Input: part model. Units: mm. Frame: model coordinates. A direction names the side the tool comes from. Give positions to 0.01 mm unless a question says otherwise; leave off trailing zeros. Loops run counter-clockwise (first coordinate to the right, second up) from the corner with the lowest first, then second, coordinate; pieces in that order, holes last. Notation, with made-up numbers: (74.25, 34.5) -> (83.25, 34.5) arc R9 cw to (83.25, 49.5) -> close; hole circle Ø8 at (-18.75, 11). An arc over 180 degrees is marked (long way). Answer as a JSON object with one key per item and string values. Group by question number.
Autodesk Inventor part; units mm, degrees
ref_plane "YZ Plane" through (0, 0, 0) normal (1, 0, 0) x (0, 1, 0)
ref_plane "XZ Plane" through (0, 0, 0) normal (0, 1, 0) x (-1, 0, 0)
ref_plane "XY Plane" through (0, 0, 0) normal (0, 0, 1) x (1, 0, 0)
sketch "Sketch1" plane through (0, 0, 0) normal (0, 1, 0) x (-1, 0, 0)
  line L0 (125, 0) -> (125, -63)
  line L1 (125, -63) -> (-4.2, -63)
  line L2 (-4.2, -63) -> (-4.2, 0)
  line L3 (-4.2, 0) -> (5.8, 0)
  line L4 (5.8, 0) -> (5.8, 40)
  line L5 (20.8, 40) -> (20.8, 0)
  line L6 (20.8, 0) -> (125, 0)
  line L7 (5.8, 40) -> (5.8, 70)
  line L8 (5.8, 70) -> (20.8, 70)
  line L9 (20.8, 70) -> (20.8, 40)
  line L10 (125, 0) -> (125, 20)
  line L11 (125, 20) -> (5.8, 20)
  line L12 (-4.2, -1.8) -> (-4.2, -60.8)
  line L13 (-4.2, 0) -> (5.8, 20)
  line L14 (125, -35.426) -> (125, -25.426)
  point P0 (20.8, 20)
  dimension "d1" = 63
  dimension "d2" = 15
  dimension "d3" = 40
  dimension "d4" = 10
  dimension "d51" = 30
  dimension "d127" = 20
  dimension "d129" = 126.9309
  dimension "d130" = 104.2
  dimension "d131" = 13.4164
extrude "Extrusion1" add sketch "Sketch1" along normal blind 2
sketch "Sketch2" plane through (0, 2, 0) normal (0, 1, 0) x (1, 0, 0)
  line L0 (-73.3, 3.3) -> (-3.3, 3.3) construction
  line L1 (-3.3, 3.3) -> (-3.3, 59.3) construction
  line L2 (-3.3, 59.3) -> (-73.3, 59.3) construction
  line L3 (-73.3, 59.3) -> (-73.3, 3.3) construction
  circle A0 centre (-73.3, 3.3) radius 1.7
  circle A1 centre (-73.3, 59.3) radius 1.7
  circle A2 centre (-3.3, 59.3) radius 1.7
  point P0 (0, 0)
  dimension "d7" = 70
  dimension "d8" = 56
  dimension "d9" = 3.3
  dimension "d11" = 3.4
  dimension "d12" = 3.4
  dimension "d13" = 3.4
  dimension "d197" = 3.3
hole "Hole1" at (-73.3, 2, -3.3) at (-73.3, 2, -59.3) at (-3.3, 2, -59.3) direction (0, -1, 0) diameter 4.4 end through all
sketch "Sketch3" plane through (0, 2, 0) normal (0, 1, 0) x (1, 0, 0)
  circle A0 centre (-3.3, 59.3) radius 2.2 construction
  circle A1 centre (-73.3, 59.3) radius 2.2 construction
  circle A2 centre (-73.3, 3.3) radius 2.2 construction
  line L0 (-20.8, -20) -> (-20.8, -70) construction
  line L1 (-5.8, -70) -> (-5.8, -20) construction
  line L2 (4.2, 0) -> (4.2, 63) construction
  line L3 (4.2, 63) -> (-125, 63) construction
  line L4 (-73.3, 3.3) -> (-3.3, 3.3) construction
  line L5 (-3.3, 3.3) -> (-3.3, 59.3) construction
  line L6 (-3.3, 38.3) -> (-38.3, 38.3) construction
  line L7 (-38.3, 38.3) -> (-38.3, 3.3) construction
  circle A3 centre (-38.3, 38.3) radius 2.2 construction
  line L8 (-20.8, -70) -> (-5.8, -70)
  line L9 (-5.8, -20) -> (4.2, 0)
  line L10 (-125, 63) -> (-125, -20)
  line L11 (-125, -20) -> (-20.8, -20)
  point P0 (0, 0)
  dimension "d24" = 35
  dimension "d25" = 35
  dimension "d26" = 4.4
hole "Hole2" at (-38.3, 2, -38.3) direction (0, -1, 0) diameter 4.4 end through all
sketch "Sketch5" plane through (0, 2, 0) normal (0, 1, 0) x (1, 0, 0)
  circle A0 centre (-38.3, 38.3) radius 2.2
  circle A1 centre (-5.5339, 15.3569) radius 2.625
  line L0 (-38.3, 38.3) -> (-5.5339, 15.3569)
  line L1 (-38.3, 38.3) -> (-38.3, 10.8789)
  point P0 (0, 0)
  dimension "d44" = 5.25
  dimension "d46" = 40
  dimension "d47" = 55
  dimension "d200" = 27.4211
extrude "Extrusion2" add sketch "Sketch5" along normal blind 15 contours A1
sketch "Sketch6" plane through (0, 2, 0) normal (0, 1, 0) x (1, 0, 0)
  line L0 (-80.8, 40.4259) -> (-55.8, 40.4259)
  line L1 (-55.8, 40.4259) -> (-55.8, 30.4259)
  line L2 (-55.8, 30.4259) -> (-80.8, 30.4259)
  line L3 (-80.8, 30.4259) -> (-80.8, 40.4259)
  circle A0 centre (-5.5339, 15.3569) radius 2.625
  circle A1 centre (-5.5339, 15.3569) radius 2.625
  line L4 (-5.5339, 15.3569) -> (-80.8, 15.3569) construction
  point P0 (0, 0)
  point P1 (-55.8, 35.4259)
  dimension "d54" = 10
  dimension "d132" = 25
  dimension "d133" = 30.4259
  dimension "d134" = 66.0957
  dimension "d206" = 80.8
extrude "Extrusion3" add sketch "Sketch6" along normal blind 15 contours L0 L1 L2 L3
sketch "Sketch7" plane through (-80.8, 2, -40.4259) normal (-1, 0, 0) x (0, 0, 1)
  line L0 (10, 2.5) -> (5, 2.5)
  line L1 (9.9999, 7.5) -> (6.9999, 7.5)
  line L2 (10, 0) -> (10, 15)
  line L3 (4.9999, 5) -> (6.9999, 5)
  line L4 (6.9999, 5) -> (6.9999, 7.5)
  line L5 (-22.5741, 0) -> (60.4259, 0)
  line L6 (7.2499, 7.5) -> (7.2499, 5)
  line L7 (7.2499, 5) -> (6.9999, 5)
  line L8 (5, 10.45) -> (10, 10.45)
  line L9 (5, 10.45) -> (5, 2.5)
  line L10 (7.2499, 7.5) -> (9.9999, 7.5)
  line L11 (10, 2.5) -> (9.9999, 7.5)
  point P0 (5, 5)
  dimension "d186" = 0.25
  dimension "d256" = 2.5
  dimension "d257" = 0.25
  dimension "d274" = 7.95
  dimension "d275" = 5
extrude "Extrusion4" cut sketch "Sketch7" against normal up to surface (25 mm away) contours L1 L4 L3 L9 L8 L2 | L6 L7 L4 L1
sketch "Sketch13" plane through (0, 2, 0) normal (0, 1, 0) x (1, 0, 0)
  point P0 (0, 0)
sketch "Sketch15" plane through (-80.8, 2, -40.4259) normal (-1, 0, 0) x (0, 0, 1)
  line L0 (10, 10.45) -> (10, 15)
  line L1 (0, 15) -> (10, 15)
  line L2 (0, 0) -> (0, 15)
  line L3 (10, 0) -> (0, 0)
  line L4 (10, 0) -> (10, 2.5)
  line L5 (5, 10.45) -> (10, 10.45)
  line L6 (5, 5) -> (5, 10.45)
  line L7 (10, 2.5) -> (9.9999, 7.5)
  line L8 (9.9999, 7.5) -> (7.2499, 7.5)
  line L9 (7.2499, 7.5) -> (7.2499, 5)
  line L10 (7.2499, 5) -> (5, 5)
  point P0 (40.4259, -2)
extrude "Extrusion9" add sketch "Sketch15" along normal up to surface (44.2 mm away)
sketch "Sketch18" plane through (0, 2, 0) normal (0, 1, 0) x (1, 0, 0)
  point P0 (0, 0)
  point P1 (-43.3, -10.4414)
  point P2 (-13.3, -35.9207)
hole "Hole4" at (-43.3, 2, 10.4414) at (-13.3, 2, 35.9207) direction (0, -1, 0) diameter 3.4 end through all
chamfer "Chamfer1" distance 50.5 distance2 44.25 1 edges at (-125, 1, 20) measured on face at (-125, 0.6667, -24.4753)
chamfer "Chamfer2" distance 44.25 distance2 22.5 1 edges at (-125, 1, -63) measured on face at (-38.8667, 1.3333, -63)
sketch "Sketch19" plane through (0, 2, 0) normal (0, 1, 0) x (1, 0, 0)
  line L0 (-125, 30.5) -> (-80.75, -20)
  line L1 (-80.75, -20) -> (-80.75, 30.4259)
  line L2 (-55.8, 30.4259) -> (-124.9351, 30.4259)
  line L3 (-124.9351, 30.4259) -> (-80.75, -20)
  line L4 (-80.75, 63.1491) -> (-125, 40.4259)
  line L5 (-125, 40.4259) -> (-80.75, 40.4259)
  line L6 (-80.75, 40.4259) -> (-80.75, 63.1491)
  line L7 (-80.75, 30.4259) -> (-124.9351, 30.4259)
  line L8 (-83.75, 27.4259) -> (-83.75, -12.0241)
  line L9 (-83.75, -12.0241) -> (-118.3176, 27.4259)
  line L10 (-118.3176, 27.4259) -> (-83.75, 27.4259)
  line L11 (-83.75, 43.4259) -> (-112.5906, 43.4259)
  line L12 (-112.5906, 43.4259) -> (-83.75, 58.2361)
  line L13 (-83.75, 58.2361) -> (-83.75, 43.4259)
  line L14 (-80.75, 0) -> (-20.75, 0)
  line L15 (-20.75, 0) -> (-20.75, 30.4259)
  line L16 (-20.75, 30.4259) -> (-80.75, 30.4259)
  line L17 (-80.75, 0) -> (-80.75, 30.4259)
  line L18 (-80.75, 27.4259) -> (-23.75, 27.4259)
  line L19 (-23.75, 27.4259) -> (-23.75, 0)
  line L20 (-65.85, 0) -> (-65.85, 27.4259)
  circle A0 centre (-73.3, 3.3) radius 2.2
  line L21 (-75.75, 54.3) -> (-3.8, 54.3)
  line L22 (-3.8, 54.3) -> (-3.8, 43.3)
  line L23 (-3.8, 43.3) -> (-75.75, 43.3)
  line L24 (-75.75, 43.3) -> (-75.75, 54.3)
  line L25 (4.2, 0) -> (4.2, 63)
  circle A1 centre (-38.3, 38.3) radius 2.2
  circle A2 centre (-73.3, 59.3) radius 2.9111
  point P0 (0, 0)
  dimension "d160" = 3
  dimension "d161" = 3
  dimension "d164" = 60
  dimension "d165" = 30.4259
  dimension "d167" = 3
  dimension "d168" = 3
  dimension "d169" = 7.45
  dimension "d176" = 5
  dimension "d177" = 8
  dimension "d178" = 5
  dimension "d179" = 5
  dimension "d312" = 49.7434
extrude "Extrusion11" cut sketch "Sketch19" against normal blind 10 contours L20 L18 L19 L14 | L8 L9 L10 | L11 L12 L13 | L21 L22 L23 L24
sketch "Sketch20" plane through (-125, 17, -30.4259) normal (0, 0, 1) x (1, 0, 0)
  line L0 (0, -4.55) -> (69.2, -4.55)
  line L1 (69.2, -4.55) -> (69.2, 0)
  line L2 (69.2, 0) -> (0, 0)
  line L3 (0, 0) -> (0, -4.55)
  point P0 (125, -17)
extrude "Extrusion12" add sketch "Sketch20" along normal blind 3
fillet "Fillet1" radius 3 2 edges at (-90.4, 17, -40.4259) (-90.4, 17, -27.4259)
sketch "Sketch21" plane through (0, 2, 0) normal (0, 1, 0) x (1, 0, 0)
  line L0 (-80.75, -20) -> (-20.8, -20)
  line L1 (-20.8, -70) -> (-5.8, -70)
  line L2 (-20.8, -20) -> (-5.8, -20)
  line L3 (-5.8, -20) -> (-5.8, -70)
  line L4 (-5.8, -70) -> (-20.8, -70)
  line L5 (-20.8, -70) -> (-20.8, -20)
  circle A0 centre (-13.3, -35.9207) radius 1.7
  point P0 (0, 0)
extrude "Extrusion13" add sketch "Sketch21" along normal blind 10
fillet "Fillet2" radius 5 1 edges at (-5.8, 12, 45)
sketch "Sketch22" plane through (-20.8, 0, 70) normal (0, 0, 1) x (1, 0, 0)
  line L0 (0, 8.6171) -> (3.5, 8)
  line L1 (3.5, 11) -> (0, 10.3829)
  line L2 (3.5, 11) -> (3.5, 8)
  line L3 (0, 0) -> (15, 0)
  line L4 (0, 0) -> (0, 12)
  line L5 (0, 10.3829) -> (0, 8.6171)
  dimension "d333" = 80
  dimension "d334" = 80
  dimension "d336" = 3
  dimension "d346" = 15
  dimension "d347" = 3.5
  dimension "d348" = 8.6171
extrude "Extrusion14" cut sketch "Sketch22" against normal blind 45
sketch "Sketch23" plane through (0, 12, 0) normal (0, 1, 0) x (1, 0, 0)
  circle A0 centre (-13.3, -35.9207) radius 1.7
  point P0 (0, 0)
hole "Hole5" at (-13.3, 12, 35.9207) direction (0, -1, 0) diameter 7 depth 6
properties part number "BasePlate"
Q1. Section A-A on x = -13.3. Return the cut outline in (y, z), then the cut area to 3 significant figures.
Q2. Pull-direction query (Z, two-part tool) for faces 4 (the face through (-71.35, 0.99, -58.28)), 5 (the face through (-90.884, 16.098, -28.281)), 6 (the face through (-20.8, 6, 45)); classes: +Z half, -Z half, draft (parallel to the pull), parting line (faces both ways), or undercut.
Q3. Section B-B on z = -9. Return the cut outline in (x, y).
Q4. Pin query (flat end, axial travel): pin 1 Ø1 at (y, z) = (1.5, -4.5) entering from -X; pin 2 Ø5.5 at (x, z) = (-38.3, -38.3) entering from -Y; pin 3 Ø1.5 at (x, z) = (-19, 31.5) entering from +Y; pin 4 Ø0.6 at (y, z) = (1, -50.5) entering from -X. Return the tip coordinate at first contact, or that it passes through.
Q5. Section D-D on y = 15.5. Return the cut outline in (x, z) (3 decimals), then the cut area to 3 significant figures.
Q6. Section C-C on x = -43.3. Return the cut outline in (y, z).
Q7. Set-up query: faces 1 (the face through (-100.79, 1.01, -7.42)), 2 (the face through (-3.03, 9.4, -14.57)), 3 (the face through (-19, 10.7, 47.8)). Return all of +Z, -Z, +X, -X, +Y, -Y with unobstructed straight access to the full face (end or side cutting, diameter ignored); none if empty.
Q8. Ray query, probe 1 along Z at (x, y) = (-73.3, 1.2); probe 2 along Z at (x, y) = (-38.3, 1.1); probe 3 along Z at (x, y) = (-13.3, 2.1). Return the intervals inside material, ascending.
Numbers:
{
 "1": {"outline": "(0, -63) -> (2, -63) -> (2, -54.3) -> (0, -54.3) -> close; (0, -43.3) -> (2, -43.3) -> (2, 20) -> (12, 20) -> (12, 32.42) -> (6, 32.42) -> (6, 34.22) -> (0, 34.22) -> close; (0, 37.62) -> (6, 37.62) -> (6, 39.42) -> (12, 39.42) -> (12, 70) -> (0, 70) -> close", "area": "682 mm²"},
 "2": {"face 4": "undercut", "face 5": "+Z half", "face 6": "draft"},
 "3": {"outline": "(-106.16, 0) -> (-102.17, 0) -> (-102.17, 2) -> (-106.16, 2) -> close; (-83.75, 0) -> (-65.85, 0) -> (-65.85, 2) -> (-83.75, 2) -> close; (-23.75, 0) -> (4.2, 0) -> (4.2, 2) -> (-23.75, 2) -> close"},
 "4": {"pin 1": "stops at x = -102.66", "pin 2": "stops at y = 0", "pin 3": "stops at y = 12", "pin 4": "stops at x = -105.92"},
 "5": {"outline": "(-125, -40.024) -> (-55.8, -40.024) -> (-55.8, -27.828) -> (-125, -27.828) -> close; circle Ø5.25 at (-5.534, -15.357)", "area": "866 mm²"},
 "6": {"outline": "(0, -63) -> (2, -63) -> (2, -54.3) -> (0, -54.3) -> close; (0, -43.3) -> (2, -43.3) -> (2, -27.43) -> (0, -27.43) -> close; (0, 0) -> (2, 0) -> (2, 8.74) -> (0, 8.74) -> close; (0, 12.14) -> (2, 12.14) -> (2, 20) -> (0, 20) -> close"},
 "7": {"face 1": "+Y, -Y", "face 2": "+Y", "face 3": "+Z"},
 "8": {"probe 1": "z = -63 to -61.5, -57.1 to -54.3, -43.3 to -5.5, -1.1 to 20", "probe 2": "z = -63 to -54.3, -43.3 to -40.5, -36.1 to -27.43, 0 to 20", "probe 3": "z = 20 to 34.22, 37.62 to 70"}
}
